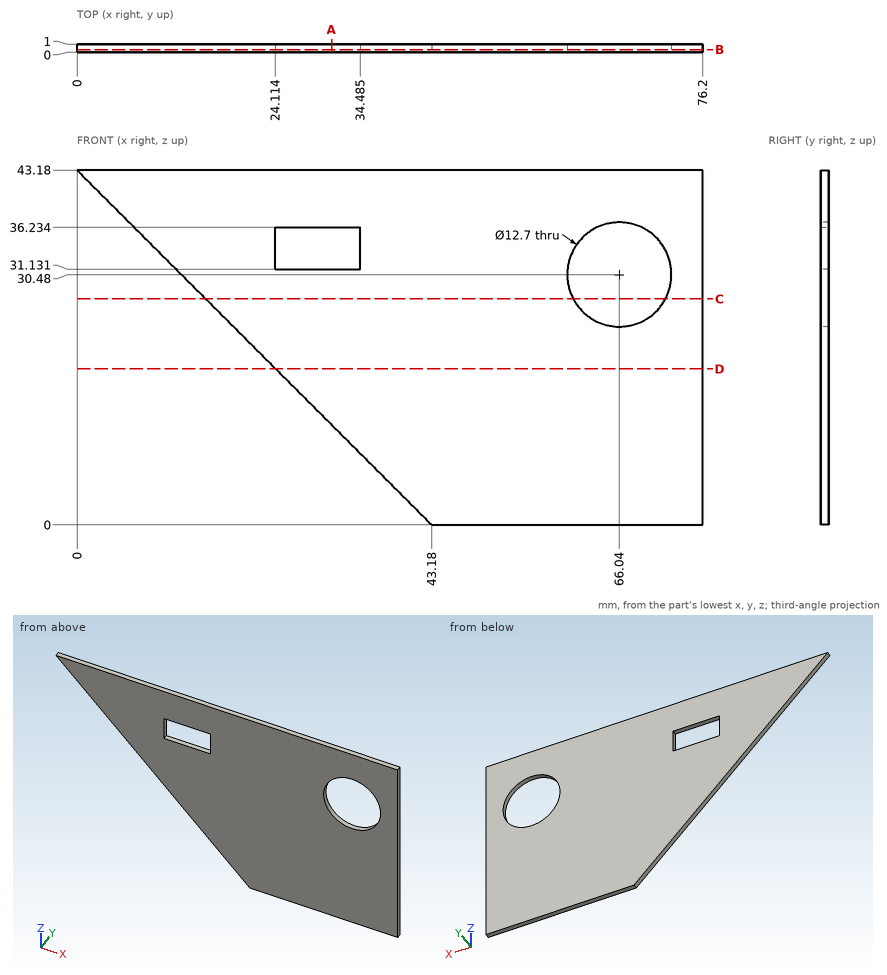
Study the drawing (mm; zero at the part's minimum x, y, z) and answer. Coordinates: 2 decimals unless noted, no trailing zeros. Loops run counter-clockwise (first coordinate to the right, second up) from the corner with the lowest first, then second, coordinate; pieces in that order, holes last. Notation, with made-up numbers: M 59,-38 L 74,-38 A34 ccw 74,-3 Z; hole C 10,-37 d5. An arc over 180 degrees is marked long. Answer in a Markdown table with one row per item. Add a question column.
1. Find section C-C, the plane z = 27.5. Write down the section's boundary in (x, y).
2. Find section B-B, the plane y = 0.3. Write down the section's boundary in (x, z) (3 decimals).
3. Find section A-A, the plane x = 31. Write down the section's boundary in (y, z), then the cut area to 3 significant figures.
4. Consider L1, parallel to Z at x = 66.04, y = 0.75; L2, parallel to X at y = 0.75, z = 35.5 (1 decimal); L3, parallel to X at y = 0.55, z = 25. Determine where each line is inside the solid, lowest interval first.
5. Find section D-D, the plane z = 19. Write down the section's boundary in (x, y).
Reported:
| question | item | result |
|---|---|---|
| 1 | outline | M 15.68,0 L 60.43,0 L 60.43,1 L 15.68,1 Z; M 71.65,0 L 76.2,0 L 76.2,1 L 71.65,1 Z |
| 2 | outline | M 0,43.18 L 43.18,0 L 76.2,0 L 76.2,43.18 Z; hole M 24.114,31.131 L 34.485,31.131 L 34.485,36.234 L 24.114,36.234 Z; hole C 66.04,30.48 d12.7 |
| 3 | outline | M 0,12.18 L 1,12.18 L 1,31.13 L 0,31.13 Z; M 0,36.23 L 1,36.23 L 1,43.18 L 0,43.18 Z |
| 3 | area | 25.9 mm^2 |
| 4 | L1 | z = 0 to 24.13, 36.83 to 43.18 |
| 4 | L2 | x = 7.7 to 24.1, 34.5 to 62.2, 69.9 to 76.2 |
| 4 | L3 | x = 18.18 to 62.83, 69.25 to 76.2 |
| 5 | outline | M 24.18,0 L 76.2,0 L 76.2,1 L 24.18,1 Z |
